from build123d import *

# Parameters (mm, degrees)
SKETCH1_W           = 228.6
SKETCH1_H           = 63.5
BOSS_EXTRUDE1_DEPTH = 6.35
SKETCH2_R           = 9.525
CUT_EXTRUDE1_DEPTH  = 7.35
LPATTERN1_COUNT     = 3
LPATTERN1_PITCH     = 82.55


with BuildPart() as part:
    # Sketch1 → Boss-Extrude1 (new body)
    with BuildSketch(Plane.XY):
        Rectangle(SKETCH1_W, SKETCH1_H)
    extrude(amount=BOSS_EXTRUDE1_DEPTH)

    # Sketch2 → Cut-Extrude1 (cut, through all)
    with BuildSketch(Plane.XY.offset(6.35)):
        with Locations((-82.55, 0)):
            Circle(SKETCH2_R)
    cut_extrude1 = extrude(amount=-CUT_EXTRUDE1_DEPTH, mode=Mode.SUBTRACT)

    # LPattern1: Cut-Extrude1 ×3
    with Locations(*[(i * LPATTERN1_PITCH, 0, 0) for i in range(1, LPATTERN1_COUNT)]):
        add(cut_extrude1, mode=Mode.SUBTRACT)


solid = part.part
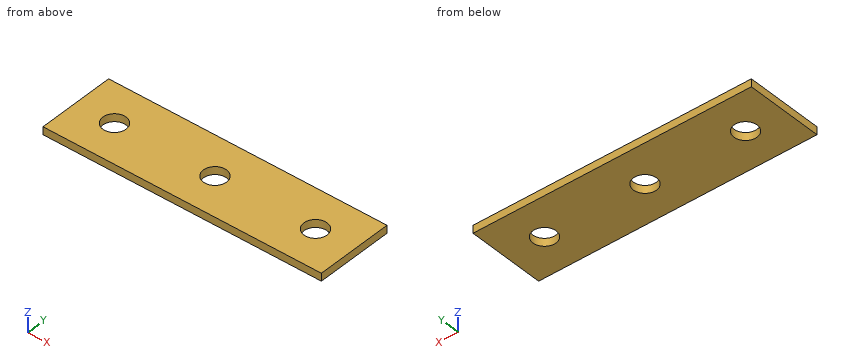
Geometry check sheet. Reference: the model listing, model coordinates, mm. Give positions to 0.01 mm unless a question says otherwise; leave off trailing zeros. Order: outer loops, then holes, each group sorted by start corner. A loop starts at its lowest first (then second) coordinate and runs counter-clockwise, first axis right, second up.
1. Sectioned sample at A-A (y = 0). Record the boundary of the cut face in (x, z) (3 decimals).
Completed:
outline: (-114.3, 0) - (-92.075, 0) - (-92.075, 6.35) - (-114.3, 6.35) - close; (-73.025, 0) - (-9.525, 0) - (-9.525, 6.35) - (-73.025, 6.35) - close; (9.525, 0) - (73.025, 0) - (73.025, 6.35) - (9.525, 6.35) - close; (92.075, 0) - (114.3, 0) - (114.3, 6.35) - (92.075, 6.35) - close
2. Depth check by flat-ended pin: pin 1 (11.5 mm diameter, centred on x = 82.55, y = 0, fed in from -Z). Enter the tip coordinate at first touch or a pass-through.
Completed:
pin 1: passes through
3. Scan lines: line 1 (Y direction, x = 82.55, z = 5.25) (3 decimals); line 2 (X direction, y = 4.5, z = 2.5); line 3 (X direction, y = -7.5, z = 1.75). Record each from-to range of solid material in increasing order.
Completed:
line 1: y = -31.75 to -9.525, 9.525 to 31.75
line 2: x = -114.3 to -90.94, -74.16 to -8.39, 8.39 to 74.16, 90.94 to 114.3
line 3: x = -114.3 to -88.42, -76.68 to -5.87, 5.87 to 76.68, 88.42 to 114.3
4. Sectioned sample at B-B (z = 4.75). Record the boundary of the cut face in (x, y) (3 decimals), then the cut area to 3 significant figures.
Completed:
outline: (-114.3, -31.75) - (114.3, -31.75) - (114.3, 31.75) - (-114.3, 31.75) - close; hole circle Ø19.05 at (-82.55, 0); hole circle Ø19.05 at (0, 0); hole circle Ø19.05 at (82.55, 0)
area: 13,700 mm2
5. Sectioned sample at C-C (x = -82.55). Record the boundary of the cut face in (y, z) (3 decimals).
Completed:
outline: (-31.75, 0) - (-9.525, 0) - (-9.525, 6.35) - (-31.75, 6.35) - close; (9.525, 0) - (31.75, 0) - (31.75, 6.35) - (9.525, 6.35) - close
